Geometry: see drawing. Coordinates: mm, zero at the bounding-box minimum. Coordinates: 2 decimals unless noted, no trailing zeros. Order: outer loops, then holes, each group sorted by start corner. A loop starts at its lowest first (then second) coordinate and runs counter-clockwise, first axis right, second up.
Item 1: Section A-A on x = 9.75. State how many separate pieces and enclosed holes the cut face has.
Item 2: Ray query, line 1 (X direction, y = 102.5, z = 1.15) (1 decimal); line 2 (X direction, y = 59, z = 1.3); line 3 (Y direction, x = 19, z = 0.75). Return the intervals inside material, ascending.
Item 3: Section B-B on y = 89.4. Return the cut outline in (x, z).
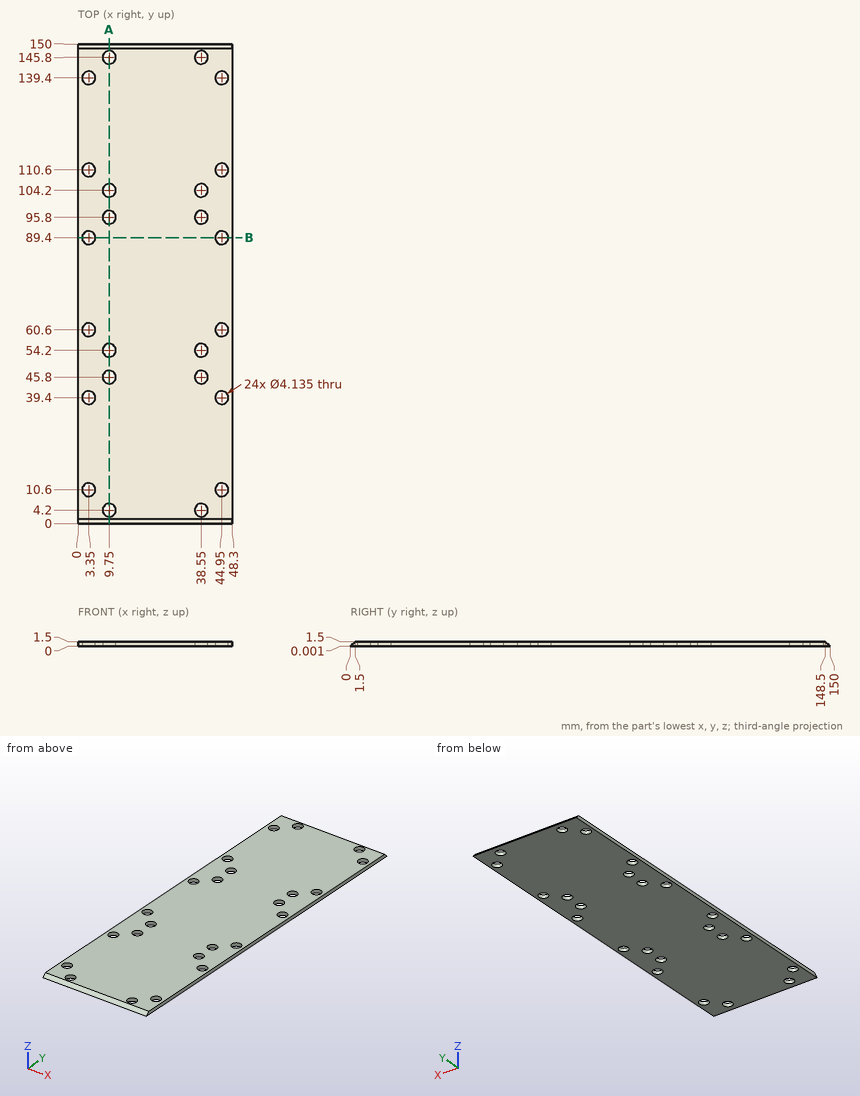
Answer list:
1. separate pieces: 7
1. enclosed holes: 0
2. line 1: x = 0 to 8.6, 10.9 to 37.4, 39.7 to 48.3
2. line 2: x = 0 to 2.04, 4.66 to 43.64, 46.26 to 48.3
2. line 3: y = 0.75 to 149.25
3. outline: (0, 0) - (1.28, 0) - (1.28, 1.5) - (0, 1.5) - close; (5.42, 0) - (42.88, 0) - (42.88, 1.5) - (5.42, 1.5) - close; (47.02, 0) - (48.3, 0) - (48.3, 1.5) - (47.02, 1.5) - close
